```python
from build123d import *

# Parameters (mm, degrees)
SKETCH1_W           = 43
SKETCH1_H           = 43
SKETCH1_R           = 13.75
SKETCH1_H_2         = 7
BOSS_EXTRUDE1_DEPTH = 60
SKETCH3_R           = 3.25
CUT_EXTRUDE5_DEPTH  = 85.038324591
CHAMFER2_SIZE       = 2.5
CUT_EXTRUDE6_START  = -38
CUT_EXTRUDE6_DEPTH  = 15
SKETCH8_W           = 10
SKETCH8_H           = 51.2
CUT_EXTRUDE8_DEPTH  = 75.012431469
FILLET2_R           = 10


with BuildPart() as part:
    # Sketch1 → Boss-Extrude1 (new body)
    # profile 1 of 3: a face of its own
    with BuildSketch(Plane.XY):
        with Locations((2.5, 2.5)):
            Rectangle(SKETCH1_W, SKETCH1_H)
        Circle(SKETCH1_R, mode=Mode.SUBTRACT)
    # profile 2 of 3: a face of its own
    with BuildSketch(Plane.XY):
        with Locations((2.5, 28.7)):
            Rectangle(SKETCH1_W, SKETCH1_H_2)
    # profile 3 of 3: a face of its own
    with BuildSketch(Plane.XY):
        Polygon((24, 24), (24, -19), (29, -19), (29, 32.2), (24, 32.2), (24, 25.2), align=None)
    extrude(amount=BOSS_EXTRUDE1_DEPTH)

    # Sketch3 → Cut-Extrude5 (cut, through all)
    with BuildSketch(Plane(origin=(0, 32.2, 0), x_dir=(1, 0, 0), z_dir=(0, 1, 0))):
        with Locations(Location((0, -50, 0), (0, 0, 270))):
            Circle(SKETCH3_R)
        with Locations(Location((0, -10, 0), (0, 0, 270))):
            Circle(SKETCH3_R)
    extrude(amount=-CUT_EXTRUDE5_DEPTH, mode=Mode.SUBTRACT)

    # Chamfer2
    chamfer2_edges = [part.edges().sort_by_distance(p)[0] for p in [
        (0, 32.2, 46.75),
        (0, 32.2, 6.75),
    ]]
    chamfer(chamfer2_edges, length=CHAMFER2_SIZE)

    # Sketch7 → Cut-Extrude6 (cut)
    with BuildSketch(Plane.XZ.offset(19).offset(CUT_EXTRUDE6_START)):
        Polygon((0, 43.533676985), (5.6, 46.766838493), (5.6, 53.233161507), (0, 56.466323015), (-5.6, 53.233161507), (-5.6, 46.766838493), align=None)
        Polygon((-5.6, 13.233161507), (0, 16.466323015), (5.6, 13.233161507), (5.6, 6.766838493), (0, 3.533676985), (-5.6, 6.766838493), align=None)
    extrude(amount=CUT_EXTRUDE6_DEPTH, mode=Mode.SUBTRACT)

    # Sketch8 → Cut-Extrude8 (cut, through all)
    with BuildSketch(Plane(origin=(0, 0, 0), x_dir=(-1, 0, 0), z_dir=(0, 0, -1))):
        with Locations((-24, 6.6)):
            Rectangle(SKETCH8_W, SKETCH8_H)
    extrude(amount=-CUT_EXTRUDE8_DEPTH, mode=Mode.SUBTRACT)


with BuildPart() as body_2:
    # of the pieces the cut leaves, the one that is kept (cut_extrude8_keep)
    add(part.part.solids().sort_by_distance((-19, 24, 0))[0])

    # Fillet2
    fillet2_edges = [body_2.edges().sort_by_distance(p)[0] for p in [
        (-19, -19, 30),
        (19, -19, 30),
    ]]
    fillet(fillet2_edges, radius=FILLET2_R)


solid = body_2.part
```
Work out the finished part from the listing and answer in its coordinate system (mm). A direction names the side the tool comes from. Round coordinates to 2 decimals unless told otherwise and drop trailing zeros. Loops run counter-clockwise (first coordinate to the right, second up) from the corner with the lowest first, then second, coordinate; pieces in that order, holes last. Notation, with made-up numbers: M 0.25,77 L 18.25,77 A11 cw 18.25,82 Z; hole C 17.5,77 d6. An arc over 180 degrees is marked long. Use CSV: the item, a comma, the result in double quotes.
Q1. Section D-D, the plane x = -8 is taken. Determine the outline of the cut face in (y, z), then the cut area to 3 significant figures.
Determined:
outline,"M -19,0 L -11.18,0 L -11.18,60 L -19,60 Z; M 11.18,0 L 24,0 L 24,60 L 11.18,60 Z"
area,"1,240 mm2"
Q2. Consider L1, parallel to Z at x = 0, y = -15.05; L2, parallel to X at y = 22, z = 50; L3, parallel to Y at x = 0, z = 45. Determine where each line is inside the solid, lowest interval first.
Determined:
L1,"0 to 6.75, 13.25 to 46.75, 53.25 to 60"
L2,"-19 to -3.25, 3.25 to 19"
L3,"-19 to -13.75, 19 to 24"
Q3. Section B-B, the plane z = 50 is taken. Determine the outline of the cut face in (x, y), then the cut area to 3 significant figures.
Determined:
outline,"M -19,-9 A10 ccw -9,-19 L -3.25,-19 L -3.25,-13.36 A13.75 cw -5.6,12.56 L -5.6,19 L -3.25,19 L -3.25,24 L -19,24 Z; M 3.25,-19 L 9,-19 A10 ccw 19,-9 L 19,24 L 3.25,24 L 3.25,19 L 5.6,19 L 5.6,12.56 A13.75 cw 3.25,-13.36 Z"
area,"866 mm2"
Q4. Section C-C, the plane z = 41.5 is taken. Determine the outline of the cut face in (x, y).
Determined:
outline,"M -19,-9 A10 ccw -9,-19 L 9,-19 A10 ccw 19,-9 L 19,24 L -19,24 Z; hole C 0,0 d27.5"
Q5. The mould has two halves that part along Y. Classify faces 3 (the cylindrical face through (0.143, 21.535, 6.753)), 4 (the flat face through (-5.6, 16, 50)), 5 (the cylindrical face through (15.99, -16.15, 30.42)): pulls with the +Y half, pulls with the -Y half, needs draft (parallel to the pull), parting line crosses it, or undercut.
Determined:
face 3,"needs draft"
face 4,"undercut"
face 5,"pulls with the -Y half"
Q6. Each of these flat-tipped pins is pushed along its axis until it touches: pin 1 (6 mm diameter, centred on x = 0, z = 10, fed in from +Y); pin 2 (1.5 mm diameter, centred on y = -12.5, z = 24.5, fed in from -X); pin 3 (2 mm diameter, centred on x = 12, z = 13.5, fed in from -Y). Where does it stop, or does it pass through?
Determined:
pin 1,"through"
pin 2,"x = -18.61"
pin 3,"y = -18.8"
Q7. Section A-A, the plane y = 0 is taken. Determine the outline of the cut face in (x, z).
Determined:
outline,"M -19,0 L -13.75,0 L -13.75,60 L -19,60 Z; M 13.75,0 L 19,0 L 19,60 L 13.75,60 Z"
Q8. A tool of negligible diameter and unlimited length cuts with its end or side. For faces 1 (the flat face through (0, -19, 30)), 2 (the flat face through (-2.839, 15.824, 45.173)), from which of +Z, -Z, +X, -X, +Y, -Y can it reach the whole face along a straight path? Write none if from no direction.
Determined:
face 1,"+Z, -Z, +X, -X, -Y"
face 2,"none"
